from build123d import *

# Parameters (mm, degrees)
SKETCH_1_R      = 5
EXTRUDE_1_DEPTH = 6


with BuildPart() as part:
    # Эскиз1 → Бобышка-Вытянуть1 (new body)
    with BuildSketch(Plane(origin=(0, 0, 0), x_dir=(1, 0, 0), z_dir=(0, 1, 0))):
        with BuildLine():
            Line((86.763576424, -13.868211788), (86.763576424, -4.868211788))
            Line((86.763576424, -4.868211788), (98.763576424, -4.868211788))
            Line((98.763576424, -4.868211788), (98.763576424, 5.131788212))
            Line((98.763576424, 5.131788212), (86.763576424, 5.131788212))
            Line((86.763576424, 5.131788212), (86.763576424, 14.131788212))
            Line((86.763576424, 14.131788212), (47.513576424, 14.131788212))
            Line((47.513576424, 14.131788212), (47.263576424, 20.231788212))
            Line((47.263576424, 20.231788212), (37.263576424, 20.231788212))
            Line((37.263576424, 20.231788212), (37.013576424, 14.131788212))
            Line((37.013576424, 14.131788212), (31.763576424, 14.131788212))
            Line((31.763576424, 14.131788212), (31.763576424, 7.331788212))
            Line((31.763576424, 7.331788212), (33.013576424, 7.331788212))
            Line((33.013576424, 7.331788212), (33.013576424, 5.131788212))
            Line((33.013576424, 5.131788212), (31.763576424, 5.131788212))
            Line((31.763576424, 5.131788212), (31.763576424, 3.631788212))
            Line((31.763576424, 3.631788212), (28.763576424, 3.631788212))
            Line((28.763576424, 3.631788212), (28.763576424, 5.131788212))
            Line((28.763576424, 5.131788212), (27.513576424, 5.131788212))
            Line((27.513576424, 5.131788212), (27.513576424, 7.331788212))
            Line((27.513576424, 7.331788212), (28.763576424, 7.331788212))
            Line((28.763576424, 7.331788212), (28.763576424, 14.131788212))
            Line((28.763576424, 14.131788212), (23.513576424, 14.131788212))
            Line((23.513576424, 14.131788212), (23.263576424, 20.231788212))
            Line((23.263576424, 20.231788212), (13.263576424, 20.231788212))
            Line((13.263576424, 20.231788212), (13.013576424, 14.131788212))
            Line((13.013576424, 14.131788212), (-12.486423576, 14.131788212))
            Line((-12.486423576, 14.131788212), (-12.736423576, 20.231788212))
            Line((-12.736423576, 20.231788212), (-22.736423576, 20.231788212))
            Line((-22.736423576, 20.231788212), (-22.986423576, 14.131788212))
            Line((-22.986423576, 14.131788212), (-28.236423576, 14.131788212))
            Line((-28.236423576, 14.131788212), (-28.236423576, 7.331788212))
            Line((-28.236423576, 7.331788212), (-26.986423576, 7.331788212))
            Line((-26.986423576, 7.331788212), (-26.986423576, 5.131788212))
            Line((-26.986423576, 5.131788212), (-28.236423576, 5.131788212))
            Line((-28.236423576, 5.131788212), (-28.236423576, 3.631788212))
            Line((-28.236423576, 3.631788212), (-31.236423576, 3.631788212))
            Line((-31.236423576, 3.631788212), (-31.236423576, 5.131788212))
            Line((-31.236423576, 5.131788212), (-32.486423576, 5.131788212))
            Line((-32.486423576, 5.131788212), (-32.486423576, 7.331788212))
            Line((-32.486423576, 7.331788212), (-31.236423576, 7.331788212))
            Line((-31.236423576, 7.331788212), (-31.236423576, 14.131788212))
            Line((-31.236423576, 14.131788212), (-36.486423576, 14.131788212))
            Line((-36.486423576, 14.131788212), (-36.736423576, 20.231788212))
            Line((-36.736423576, 20.231788212), (-46.736423576, 20.231788212))
            Line((-46.736423576, 20.231788212), (-46.986423576, 14.131788212))
            Line((-46.986423576, 14.131788212), (-86.236423576, 14.131788212))
            Line((-86.236423576, 14.131788212), (-86.236423576, 5.131788212))
            Line((-86.236423576, 5.131788212), (-98.236423576, 5.131788212))
            Line((-98.236423576, 5.131788212), (-98.236423576, -4.868211788))
            Line((-98.236423576, -4.868211788), (-86.236423576, -4.868211788))
            Line((-86.236423576, -4.868211788), (-86.236423576, -13.868211788))
            Line((-86.236423576, -13.868211788), (-77.236423576, -13.868211788))
            Line((-77.236423576, -13.868211788), (-77.236423576, -10.145058633))
            ThreePointArc((-77.236423576, -10.145058633), (-69.736423576, 7.581788212), (-62.236423576, -10.145058633))
            Line((-62.236423576, -10.145058633), (-62.236423576, -13.868211788))
            Line((-62.236423576, -13.868211788), (-46.986423576, -13.868211788))
            Line((-46.986423576, -13.868211788), (-46.736423576, -19.968211788))
            Line((-46.736423576, -19.968211788), (-36.736423576, -19.968211788))
            Line((-36.736423576, -19.968211788), (-36.486423576, -13.868211788))
            Line((-36.486423576, -13.868211788), (-31.236423576, -13.868211788))
            Line((-31.236423576, -13.868211788), (-31.236423576, -7.068211788))
            Line((-31.236423576, -7.068211788), (-32.486423576, -7.068211788))
            Line((-32.486423576, -7.068211788), (-32.486423576, -4.868211788))
            Line((-32.486423576, -4.868211788), (-31.236423576, -4.868211788))
            Line((-31.236423576, -4.868211788), (-31.236423576, -3.368211788))
            Line((-31.236423576, -3.368211788), (-28.236423576, -3.368211788))
            Line((-28.236423576, -3.368211788), (-28.236423576, -4.868211788))
            Line((-28.236423576, -4.868211788), (-26.986423576, -4.868211788))
            Line((-26.986423576, -4.868211788), (-26.986423576, -7.068211788))
            Line((-26.986423576, -7.068211788), (-28.236423576, -7.068211788))
            Line((-28.236423576, -7.068211788), (-28.236423576, -13.868211788))
            Line((-28.236423576, -13.868211788), (-22.986423576, -13.868211788))
            Line((-22.986423576, -13.868211788), (-22.736423576, -19.968211788))
            Line((-22.736423576, -19.968211788), (-12.736423576, -19.968211788))
            Line((-12.736423576, -19.968211788), (-12.486423576, -13.868211788))
            Line((-12.486423576, -13.868211788), (13.013576424, -13.868211788))
            Line((13.013576424, -13.868211788), (13.263576424, -19.968211788))
            Line((13.263576424, -19.968211788), (23.263576424, -19.968211788))
            Line((23.263576424, -19.968211788), (23.513576424, -13.868211788))
            Line((23.513576424, -13.868211788), (28.763576424, -13.868211788))
            Line((28.763576424, -13.868211788), (28.763576424, -7.068211788))
            Line((28.763576424, -7.068211788), (27.513576424, -7.068211788))
            Line((27.513576424, -7.068211788), (27.513576424, -4.868211788))
            Line((27.513576424, -4.868211788), (28.763576424, -4.868211788))
            Line((28.763576424, -4.868211788), (28.763576424, -3.368211788))
            Line((28.763576424, -3.368211788), (31.763576424, -3.368211788))
            Line((31.763576424, -3.368211788), (31.763576424, -4.868211788))
            Line((31.763576424, -4.868211788), (33.013576424, -4.868211788))
            Line((33.013576424, -4.868211788), (33.013576424, -7.068211788))
            Line((33.013576424, -7.068211788), (31.763576424, -7.068211788))
            Line((31.763576424, -7.068211788), (31.763576424, -13.868211788))
            Line((31.763576424, -13.868211788), (37.013576424, -13.868211788))
            Line((37.013576424, -13.868211788), (37.263576424, -19.968211788))
            Line((37.263576424, -19.968211788), (47.263576424, -19.968211788))
            Line((47.263576424, -19.968211788), (47.513576424, -13.868211788))
            Line((47.513576424, -13.868211788), (62.763576424, -13.868211788))
            Line((62.763576424, -13.868211788), (62.763576424, -10.145058633))
            ThreePointArc((62.763576424, -10.145058633), (70.263576424, 7.581788212), (77.763576424, -10.145058633))
            Line((77.763576424, -10.145058633), (77.763576424, -13.868211788))
            Line((77.763576424, -13.868211788), (86.763576424, -13.868211788))
        make_face()
        with Locations((0.263576424, -2.868211788)):
            Circle(SKETCH_1_R, mode=Mode.SUBTRACT)
        with BuildLine():
            Line((-8.221704951, -9.232172819), (-6.100384607, -7.110852475))
            ThreePointArc((-6.100384607, -7.110852475), (-3.979064264, -7.110852475), (-3.979064264, -9.232172819))
            Line((-3.979064264, -9.232172819), (-6.100384607, -11.353493162))
            ThreePointArc((-6.100384607, -11.353493162), (-8.221704951, -11.353493162), (-8.221704951, -9.232172819))
        make_face(mode=Mode.SUBTRACT)
        with BuildLine():
            Line((-6.100384607, 5.617069586), (-3.979064264, 3.495749242))
            ThreePointArc((-3.979064264, 3.495749242), (-3.979064264, 1.374428899), (-6.100384607, 1.374428899))
            Line((-6.100384607, 1.374428899), (-8.221704951, 3.495749242))
            ThreePointArc((-8.221704951, 3.495749242), (-8.221704951, 5.617069586), (-6.100384607, 5.617069586))
        make_face(mode=Mode.SUBTRACT)
        with BuildLine():
            Line((8.748857798, -9.232172819), (6.627537454, -7.110852475))
            ThreePointArc((6.627537454, -7.110852475), (4.506217111, -7.110852475), (4.506217111, -9.232172819))
            Line((4.506217111, -9.232172819), (6.627537454, -11.353493162))
            ThreePointArc((6.627537454, -11.353493162), (8.748857798, -11.353493162), (8.748857798, -9.232172819))
        make_face(mode=Mode.SUBTRACT)
        with BuildLine():
            Line((6.627537454, 5.617069586), (4.506217111, 3.495749242))
            ThreePointArc((4.506217111, 3.495749242), (4.506217111, 1.374428899), (6.627537454, 1.374428899))
            Line((6.627537454, 1.374428899), (8.748857798, 3.495749243))
            ThreePointArc((8.748857798, 3.495749243), (8.748857798, 5.617069586), (6.627537454, 5.617069586))
        make_face(mode=Mode.SUBTRACT)
    extrude(amount=EXTRUDE_1_DEPTH)


solid = part.part
The listing builds one solid part. Answer for the finished solid, in the listing's coordinates (mm). A direction names the side the tool comes from. Round coordinates to 2 decimals unless told otherwise and drop trailing zeros. Write each loop counter-clockwise with the first axis right and the second up, starting at its lowest first coordinate (ties: lowest second). Pieces come first, ordered by that corner, then holes. Notation, with made-up numbers: (14.5, 12) - (40.5, 12) arc R21 cw to (40.5, 35) - close; hole circle Ø1 at (32.5, 17). An arc over 180 degrees is marked (long way). Use one line per item in the form item = value. Start each with the question number.
Item 1: A tool of negligible diameter and unlimited length cuts with its end or side. For faces 1 (the flat face through (-86.236, 3, 9)), 2 (the flat face through (23.387, 2.958, 16.961)), 3 (the flat face through (0, 3, -14.132)), from which of +Z, -Z, +X, -X, +Y, -Y can it reach the whole face along a straight path? Write none if from no direction.
Item 2: A cutting plane is placed at C-C (y = 2.35). Give the number of separate pieces and of enclosed holes in the cut face, plus the area to 3 significant figures.
Item 3: A cutting plane is placed at A-A (z = -12). Write down the section's boundary in (x, y).
Item 4: Find the intervals of material crossed by line 1 (X direction, y = 1.3, z = -11.5); line 2 (X direction, y = 5.25, z = 13); line 3 (X direction, y = 4.7, z = -15), in increasing order. Write a range as [from, to].
Item 5: Flat-ended cylindrical pins translate along their axes: pin 1 Ø3.5 at (x, y) = (-30, 3.5) entering from +Z; pin 2 Ø0.7 at (y, z) = (1.5, 6.5) entering from -X; pin 3 Ø1.8 at (x, y) = (-93, 2.5) entering from -Z. Find the tip coordinate at first contact, or state that the pin passes through.
Item 6: A cutting plane is placed at B-B (x = -10.5). Write down the section's boundary in (y, z).
Item 7: A cutting plane is placed at D-D (x = -71). Write down the section's boundary in (y, z), plus the area to 3 significant figures.
The answers:
q1.face_1 = +Z, -X, +Y, -Y
q1.face_2 = +Z, +Y, -Y
q1.face_3 = -Z, +Y, -Y
q2.separate_pieces = 1
q2.enclosed_holes = 5
q2.area = 4,560 mm^2
q3.outline = (-86.24, 0) - (-31.24, 0) - (-31.24, 6) - (-86.24, 6) - close; (-28.24, 0) - (28.76, 0) - (28.76, 6) - (-28.24, 6) - close; (31.76, 0) - (86.76, 0) - (86.76, 6) - (31.76, 6) - close
q4.line_1 = [-86.24, -31.24], [-28.24, 28.76], [31.76, 86.76]
q4.line_2 = [-86.24, -77.24], [-62.24, -31.24], [-28.24, 28.76], [31.76, 62.76], [77.76, 86.76]
q4.line_3 = [-46.95, -36.52], [-22.95, -12.52], [13.05, 23.48], [37.05, 47.48]
q5.pin_1 = 13.87
q5.pin_2 = -86.24
q5.pin_3 = -5.13
q6.outline = (0, -14.13) - (6, -14.13) - (6, 13.87) - (0, 13.87) - close
q7.outline = (0, -14.13) - (6, -14.13) - (6, -7.51) - (0, -7.51) - close
q7.area = 39.8 mm^2
